from build123d import *

# Parameters (mm, degrees)
SKETCH1_R           = 3.5685
SKETCH1_W           = 3
SKETCH1_H           = 5
BOSS_EXTRUDE1_DEPTH = 3
FILLET1_R           = 5


with BuildPart() as part:
    # Sketch1 → Boss-Extrude1 (new body)
    with BuildSketch(Plane(origin=(0, 0, 0), x_dir=(1, 0, 0), z_dir=(0, 1, 0))):
        Polygon((-21.821592901, -5), (-21.821592901, 10), (5.178407099, 10), (5.178407099, 5), (8.178407099, 5), (8.178407099, 0), (5.178407099, 0), (5.178407099, -5), align=None)
        with Locations((-9.121592901, 2.5)):
            Circle(SKETCH1_R, mode=Mode.SUBTRACT)
        with Locations((-16.621592901, 2.5)):
            Rectangle(SKETCH1_W, SKETCH1_H, mode=Mode.SUBTRACT)
        with Locations((-1.621592901, 2.5)):
            Rectangle(SKETCH1_W, SKETCH1_H, mode=Mode.SUBTRACT)
    extrude(amount=BOSS_EXTRUDE1_DEPTH)

    # Fillet1
    fillet1_edges = [part.edges().sort_by_distance(p)[0] for p in [
        (-21.821592901, 1.5, 5),
        (-21.821592901, 1.5, -10),
    ]]
    fillet(fillet1_edges, radius=FILLET1_R)


solid = part.part
For this review, take the finished solid that the model builds, in its own axes (mm). A direction names the side the tool comes from. Coordinates: 2 decimals unless noted, no trailing zeros. Loops run counter-clockwise (first coordinate to the right, second up) from the corner with the lowest first, then second, coordinate; pieces in that order, holes last. Notation, with made-up numbers: (87, 31) - (144, 31) arc R21 cw to (144, 63) - close; hole circle Ø11 at (56, -39). An arc over 180 degrees is marked (long way). Return JSON: item names as keys, results as strings.
Item 1: For line 1 (X direction, y = 2.2, z = -2.5); line 2 (Z direction, x = -1, y = 0.75); line 3 (X direction, y = 1, z = -3.5), list the stretches that pass through material, from the lowest coordinate up.
Determined:
{"line 1": "x = -21.82 to -18.12, -15.12 to -12.69, -5.55 to -3.12, -0.12 to 8.18", "line 2": "z = -10 to -5, 0 to 5", "line 3": "x = -21.82 to -18.12, -15.12 to -12.55, -5.7 to -3.12, -0.12 to 8.18"}
Item 2: Take a section at A-A (z = -2.5). Give the boundary of the cut face in (x, y).
Determined:
{"outline": "(-21.82, 0) - (-18.12, 0) - (-18.12, 3) - (-21.82, 3) - close; (-15.12, 0) - (-12.69, 0) - (-12.69, 3) - (-15.12, 3) - close; (-5.55, 0) - (-3.12, 0) - (-3.12, 3) - (-5.55, 3) - close; (-0.12, 0) - (8.18, 0) - (8.18, 3) - (-0.12, 3) - close"}
Item 3: Mouldability with a two-part tool opening along Z and no side actions: class faces 4 (the flat face through (5.178, 1, -8)), 5 (the flat face through (-6, 1, -10)), 6 (the flat face through (-18.122, 1, -2)) as pulls with the +Z half, pulls with the -Z half, needs draft (parallel to the pull), parting line crosses it, or undercut.
Determined:
{"face 4": "needs draft", "face 5": "pulls with the -Z half", "face 6": "undercut"}
Item 4: For faces 1 (the flat face through (-7, 0, -6)), 2 (the flat face through (-2, 1, 0)), 3 (the flat face through (5.178, 1, 2)), list the 3-axis set-ups (+Z, -Z, +X, -X, +Y, -Y) from which the entire face can be reached by the end or side of a thin tool; tool diameter is ignored.
Determined:
{"face 1": "+Z, -Z, +X, -X, -Y", "face 2": "+Y, -Y", "face 3": "+Z, +X, +Y, -Y"}
Item 5: Take a section at D-D (z = 2.5). Give the boundary of the cut face in (x, y), then the cut area to 3 significant figures.
Determined:
{"outline": "(-21.15, 0) - (5.18, 0) - (5.18, 3) - (-21.15, 3) - close", "area": "79.0 mm2"}
Item 6: Insertion check: pin 1 (0.9 mm diameter, centred on y = 1, z = -8.5, fed in from +X). The pin has a flat end and moves straight along its axis. Give the tip position at first contact, or say it passes through.
Determined:
{"pin 1": "stops at x = 5.18"}
Item 7: Take a section at C-C (x = 5.75). Give the boundary of the cut face in (y, z), then the cut area to 3 significant figures.
Determined:
{"outline": "(0, -5) - (3, -5) - (3, 0) - (0, 0) - close", "area": "15.0 mm2"}
Item 8: Take a section at B-B (y = 0.45). Give the boundary of the cut face in (x, z).
Determined:
{"outline": "(-21.82, -5) arc R5 ccw to (-16.82, -10) - (5.18, -10) - (5.18, -5) - (8.18, -5) - (8.18, 0) - (5.18, 0) - (5.18, 5) - (-16.82, 5) arc R5 ccw to (-21.82, 0) - close; hole (-18.12, -5) - (-15.12, -5) - (-15.12, 0) - (-18.12, 0) - close; hole circle Ø7.14 at (-9.12, -2.5); hole (-3.12, -5) - (-0.12, -5) - (-0.12, 0) - (-3.12, 0) - close"}
